The model under review builds one solid part; all positions refer to its coordinate system, in mm. Face numbers are marked on the shaded views. A direction names the side the tool comes from. Give positions to 0.01 mm unless a question says otherwise; leave off trailing zeros. Loops run counter-clockwise (first coordinate to the right, second up) from the corner with the lowest first, then second, coordinate; pieces in that order, holes last. Notation, with made-up numbers: M 22.25,64.5 L 74.25,64.5 A21 ccw 74.25,84.5 Z; hole C 73.25,19.25 d11. An arc over 180 degrees is marked long. Return JSON: item names as keys, results as strings.
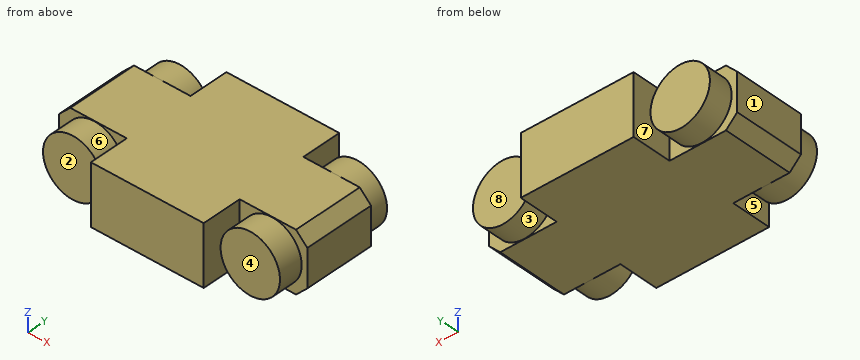
Autodesk Inventor part; units mm, degrees
ref_plane "YZ Plane" through (0, 0, 0) normal (1, 0, 0) x (0, 1, 0)
ref_plane "XZ Plane" through (0, 0, 0) normal (0, 1, 0) x (-1, 0, 0)
ref_plane "XY Plane" through (0, 0, 0) normal (0, 0, 1) x (1, 0, 0)
sketch "Sketch4" plane through (0, 0, 0) normal (0, 0, 1) x (1, 0, 0)
  line L0 (75, -100) -> (-75, -100)
  line L1 (-75, -100) -> (-75, 100)
  line L2 (-75, 100) -> (75, 100)
  line L3 (75, 100) -> (75, -100)
  line L4 (75, -100) -> (-75, 100) construction
  line L5 (-75, -100) -> (75, 100) construction
  line L6 (165, -47) -> (-165, -47)
  line L7 (-165, -47) -> (-165, 47)
  line L8 (-165, 47) -> (165, 47)
  line L9 (165, 47) -> (165, -47)
  line L10 (165, -47) -> (-165, 47) construction
  line L11 (-165, -47) -> (165, 47) construction
  point P0 (0, 0)
  point P1 (0, 0)
  point P2 (0, 0)
  point P3 (75, 47)
  point P4 (-75, 47)
  point P5 (-75, -47)
  point P6 (75, -47)
  dimension "d17" = 94
  dimension "d18" = 330
  dimension "d19" = 150
  dimension "d20" = 200
extrude "Extrusion4" add sketch "Sketch4" along normal mid plane 80
sketch "Sketch5" plane through (0, 0, 0) normal (0, 1, 0) x (-1, 0, 0)
  circle A0 centre (-118, 0) radius 39.5
  circle A1 centre (118, 0) radius 39.5
  line L0 (75, 40) -> (-75, 40) construction
  line L1 (0, 40) -> (0, -40) construction
  line L2 (-75, -40) -> (75, -40) construction
  line L3 (-165, -40) -> (-165, 40) construction
  line L4 (-165, 0) -> (165, 0) construction
  line L5 (165, -40) -> (165, 40) construction
  circle A2 centre (-118, 0) radius 31.5
  circle A3 centre (118, 0) radius 31.5
  line L6 (-150, 40) -> (-165, 25)
  line L7 (-165, -25) -> (-150, -40)
  line L8 (-165, -40) -> (-75, -40)
  line L9 (165, 40) -> (75, 40)
  line L10 (150, 40) -> (165, 25)
  line L11 (165, -25) -> (150, -40)
  line L12 (-75, 40) -> (-165, 40)
  line L13 (75, -40) -> (165, -40)
  line L14 (-165, 40) -> (-165, -40)
  line L15 (165, 40) -> (165, -40)
  point P0 (0, 0)
  dimension "d23" = 79
  dimension "d24" = 236
  dimension "d39" = 63
  dimension "d42" = 15
  dimension "d43" = 45
extrude "Extrusion5" add sketch "Sketch5" against normal blind 32 from surface at -47 contours A0 | A1 | A2 | A3
sketch "Sketch6" plane through (0, 0, 0) normal (0, 0, 1) x (1, 0, 0)
  line L0 (142, 25) -> (-142, 25)
  line L1 (-142, 25) -> (-142, -25)
  line L2 (-142, -25) -> (142, -25)
  line L3 (142, -25) -> (142, 25)
  line L4 (142, 25) -> (-142, -25) construction
  line L5 (-142, 25) -> (142, -25) construction
  line L6 (-65, 90) -> (65, 90)
  line L7 (65, 90) -> (65, -90)
  line L8 (65, -90) -> (-65, -90)
  line L9 (-65, -90) -> (-65, 90)
  line L10 (-65, 90) -> (65, -90) construction
  line L11 (65, 90) -> (-65, -90) construction
  line L12 (75, -100) -> (-75, -100)
  line L13 (-75, 47) -> (-75, 100)
  line L14 (-165, -47) -> (-165, 47)
  line L15 (-75, -47) -> (-165, -47)
  point P0 (0, 0)
  point P1 (-65, -25)
  point P2 (65, -25)
  point P3 (65, 25)
  point P4 (-65, 25)
  dimension "d27" = 10
  dimension "d28" = 10
  dimension "d29" = 23
  dimension "d30" = 22
extrude "Extrusion6" cut sketch "Sketch6" along normal mid plane 60
extrude "Extrusion8" cut sketch "Sketch5" against normal through all both and the other way through all contours L7 L8 L14 | L6 L14 L12 | L15 L10 L9 | L15 L13 L11
mirror "Mirror1" about plane through (0, 0, 0) normal (0, 1, 0) of "Extrusion5"
properties part number "body_inventor"
1) The part is to be moulded in two halves that separate along X. For the marked faces 1, 2 and 3, say which applies: released by +X, released by -X, zero draft, split by the parting line, or undercut.
From the geometry:
{"face 1": "released by -X", "face 2": "zero draft", "face 3": "undercut"}
2) Consider section D-D on x = -7. Write out the cut boundary in (y, z).
From the geometry:
{"outline": "M -100,-40 L 100,-40 L 100,40 L -100,40 Z; hole M -90,-30 L 90,-30 L 90,30 L -90,30 Z"}
3) Consider section A-A on y = 58. Write out the cut boundary in (x, z), then the cut area to 3 significant figures.
From the geometry:
{"outline": "C -118,0 d79; M -75,-40 L 75,-40 L 75,40 L -75,40 Z; C 118,0 d79; hole M -65,-30 L 65,-30 L 65,30 L -65,30 Z", "area": "14,000 mm²"}
4) Wall thickness on L1, parallel to X at y = 85, z = 4; L2, parallel to Z at x = -46, y = 75; L3, parallel to X at y = 21.5, z = -15.5: over which ranges is each line inside the solid? List them lowest first. Write a range as from..to.
From the geometry:
{"L1": "-75..-65, 65..75", "L2": "-40..-30, 30..40", "L3": "-165..-142, 142..165"}
5) Insertion check: pin 1 (1.5 mm diameter, centred on y = -28.5, z = 29.5, fed in from -X); pin 2 (16 mm diameter, centred on y = 67.5, z = -15.5, fed in from +X); pin 3 (18 mm diameter, centred on x = -99.5, z = 14.5, fed in from +Y). Each pin has a flat end and moves straight along its axis. Give the tip position at first contact, or say it passes through.
From the geometry:
{"pin 1": "x = -161.25", "pin 2": "x = 156.78", "pin 3": "y = 79"}
6) Consider section C-C on y = -2. Write out the cut boundary in (x, z), then the cut area to 3 significant figures.
From the geometry:
{"outline": "M -165,-25 L -150,-40 L 150,-40 L 165,-25 L 165,25 L 150,40 L -150,40 L -165,25 Z; hole M -142,-30 L 142,-30 L 142,30 L -142,30 Z", "area": "8,910 mm²"}
7) Tool access review of the marked faces 4, 5, 6, 7 and 8: name each direction out of +Z, -Z, +X, -X, +Y, -Y from which nothing blocks a thin tool from reaching the whole face with its end or side.
From the geometry:
{"face 4": "+Z, -Z, +X, -Y", "face 5": "+Z, -Z, -Y", "face 6": "-Y", "face 7": "+Z, -Z, +Y", "face 8": "+Z, -Z, +X, +Y"}
8) Consider section B-B on x = 118. Write out the cut boundary in (y, z), then the cut area to 3 significant figures.
From the geometry:
{"outline": "M -79,-39.5 L -47,-39.5 L -47,-40 L 47,-40 L 47,-39.5 L 79,-39.5 L 79,39.5 L 47,39.5 L 47,40 L -47,40 L -47,39.5 L -79,39.5 Z; hole M -25,-30 L 25,-30 L 25,30 L -25,30 Z", "area": "9,580 mm²"}
